Part print with two shaded views. Sizes in mm from the minimum x, y, z corner. A direction names the side the tool comes from. Give positions to 0.01 mm unless a question says otherwise; leave off trailing zeros. Order: outer loops, then holes, each group sorted by start corner. A loop starts at its lowest first (then second) coordinate and runs counter-clockwise, first axis right, second up. Notation, with made-up numbers: M -2,-28.75 L 14,-28.75 A13 cw 14,-20.75 Z; hole C 39,50.5 d6. An arc over 180 degrees is marked long. Return JSON: item names as keys, results as strings.
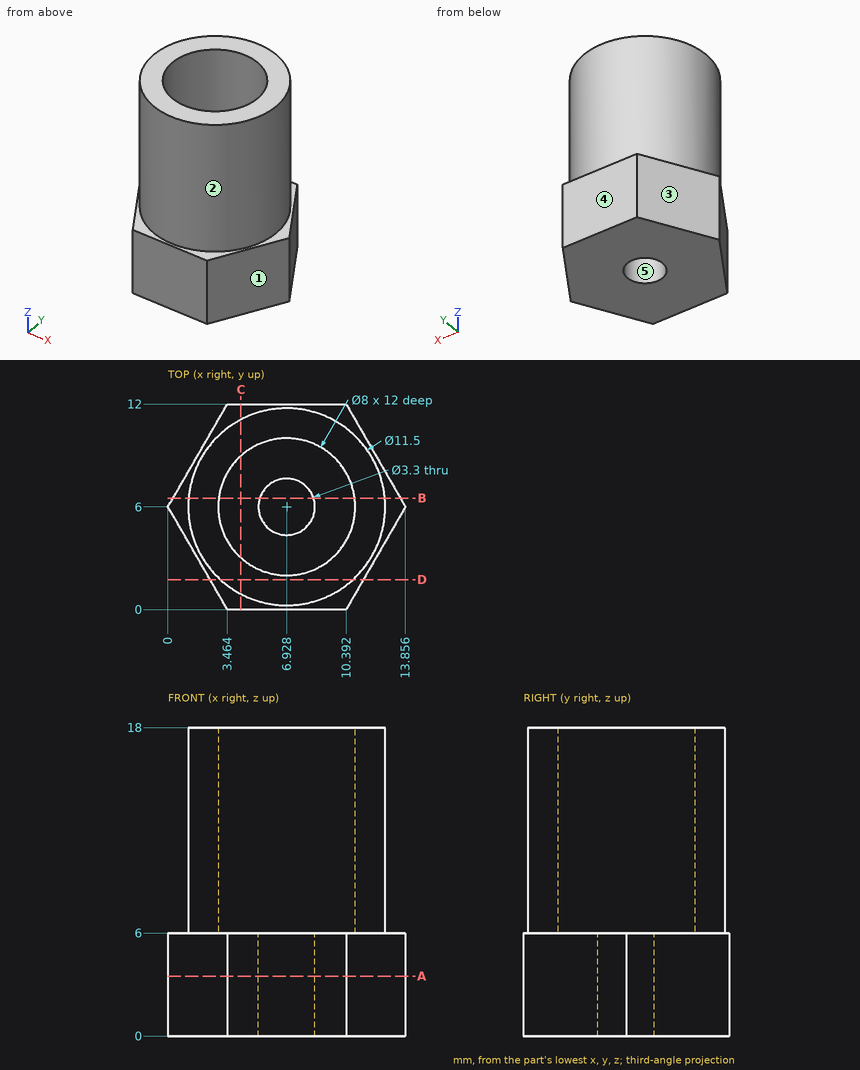
Q1. Band-saw the part on D-D (y = 1.75). Give the cut face in (x, z) (1 decimal), then the cut area to 3 significant figures.
Established:
{"outline": "M 2.5,0 L 11.4,0 L 11.4,6 L 10.8,6 L 10.8,18 L 3.1,18 L 3.1,6 L 2.5,6 Z", "area": "147 mm²"}
Q2. Two-plate mould, pull along X, no slides. Class the marked faces 3, 4 and 5: +X half, -X half, draft (parallel to the pull), parting line (faces both ways), or undercut.
Established:
{"face 3": "-X half", "face 4": "draft", "face 5": "undercut"}
Q3. Probe line 1 along Y through (x, z) = (7, 10.75); line 2 along Z through (x, y) = (7.25, 3.75); line 3 along X through (y, z) = (6.5, 4.25) (1 decimal). List the from-to ranges inside material, lowest first.
Established:
{"line 1": "y = 0.25 to 2, 10 to 11.75", "line 2": "z = 0 to 6", "line 3": "x = 0.3 to 5.4, 8.5 to 13.6"}
Q4. 3-axis set-ups, long thin cutter, end or side, ignore diameter. For the marked faces 1 and 2: which of +Z, -Z, +X, -X, +Y, -Y reach the whole face in a straight line?
Established:
{"face 1": "+Z, -Z, +X, -Y", "face 2": "+Z"}
Q5. Band-saw the part on A-A (z = 3.5). Give the cut face in (x, y).
Established:
{"outline": "M 0,6 L 3.46,0 L 10.39,0 L 13.86,6 L 10.39,12 L 3.46,12 Z; hole C 6.93,6 d3.3"}
Q6. Pin check, flat tips, straight feed: pin 1 (4 mm diameter, centred on x = 6.5, y = 6, fed in from +Z); pin 2 (4 mm diameter, centred on y = 3, z = 10.5, fed in from -X); pin 3 (2 mm diameter, centred on y = 6.5, z = 3, fed in from -X). Stop position of each tip, or through.
Established:
{"pin 1": "stops at z = 6", "pin 2": "stops at x = 1.27", "pin 3": "stops at x = 0"}
Q7. Band-saw the part on C-C (x = 4.25). Give the cut face in (y, z).
Established:
{"outline": "M 0,0 L 12,0 L 12,6 L 11.09,6 L 11.09,18 L 8.97,18 L 8.97,6 L 3.03,6 L 3.03,18 L 0.91,18 L 0.91,6 L 0,6 Z"}
Q8. Band-saw the part on B-B (y = 6.5). Give the cut face in (x, z) (1 decimal).
Established:
{"outline": "M 0.3,0 L 5.4,0 L 5.4,6 L 3,6 L 3,18 L 1.2,18 L 1.2,6 L 0.3,6 Z; M 8.5,0 L 13.6,0 L 13.6,6 L 12.7,6 L 12.7,18 L 10.9,18 L 10.9,6 L 8.5,6 Z"}
